from build123d import *

# Parameters (mm, degrees)
SKETCH1_W           = 45.5
SKETCH1_H           = 28.5
BOSS_EXTRUDE1_DEPTH = 14
SKETCH2_R           = 8
CUT_EXTRUDE1_DEPTH  = 30
SKETCH3_R           = 11.1
CUT_EXTRUDE2_DEPTH  = 26
SKETCH4_W           = 9.997259543
SKETCH4_H           = 22.5
CUT_EXTRUDE3_DEPTH  = 56.484231994


with BuildPart() as part:
    # Sketch1 → Boss-Extrude1 (new body)
    with BuildSketch(Plane.XY):
        with Locations((22.75, 14.25)):
            Rectangle(SKETCH1_W, SKETCH1_H)
    extrude(amount=BOSS_EXTRUDE1_DEPTH)

    # Sketch2 → Cut-Extrude1 (cut)
    with BuildSketch(Plane(origin=(0, 28.5, 0), x_dir=(1, 0, 0), z_dir=(0, 1, 0))):
        with Locations((22.75, 0)):
            Circle(SKETCH2_R)
    extrude(amount=-CUT_EXTRUDE1_DEPTH, mode=Mode.SUBTRACT)

    # Sketch3 → Cut-Extrude2 (cut)
    with BuildSketch(Plane.XZ):
        with Locations((22.75, 0)):
            Circle(SKETCH3_R)
    extrude(amount=-CUT_EXTRUDE2_DEPTH, mode=Mode.SUBTRACT)

    # Sketch4 → Cut-Extrude3 (cut, through all)
    with BuildSketch(Plane(origin=(45.5, 0, 0), x_dir=(0, 0, -1), z_dir=(1, 0, 0))):
        with Locations((-4.998629772, 14.75)):
            Rectangle(SKETCH4_W, SKETCH4_H)
    extrude(amount=-CUT_EXTRUDE3_DEPTH, mode=Mode.SUBTRACT)


solid = part.part
The listing builds one solid part. Answer for the finished solid, in the listing's coordinates (mm). A direction names the side the tool comes from. Give positions to 0.01 mm unless a question says otherwise; leave off trailing zeros. Loops run counter-clockwise (first coordinate to the right, second up) from the corner with the lowest first, then second, coordinate; pieces in that order, holes last. Notation, with made-up numbers: M 33,25 L 79,25 A15 ccw 79,50 Z; hole C 0.5,25 d3. An arc over 180 degrees is marked long. Answer as CSV lines item,"result".
Item 1: The part is cut by section B-B (x = 8). Give the vertices of the cut face in (y, z), and give its area (3 significant figures).
Values follow:
outline,"M 0,0 L 3.5,0 L 3.5,10 L 26,10 L 26,0 L 28.5,0 L 28.5,14 L 0,14 Z"
area,"174 mm^2"
Item 2: Which of the six approach directions +Z, -Z, +X, -X, +Y, -Y give full straight-line access (tool end or side, diameter ignored) to faces 1 (the flat face through (39, 3.5, 5)), 2 (the flat face through (0, 14, 12))?
Values follow:
face 1,"-Z, +X, -X"
face 2,"+Z, -Z, -X, +Y, -Y"
Item 3: Straight lines are drawn through the part: line 1 along Y through (x, z) = (7.5, 6.75); line 2 along X through (y, z) = (3.25, 9.25); line 3 along Z through (x, y) = (37, 16). For each, find the intervals that lie inside material, in ascending order. Write a range as [from, to].
Values follow:
line 1,"y = [0, 3.5], [26, 28.5]"
line 2,"x = [0, 16.61], [28.89, 45.5]"
line 3,"z = [10, 14]"
Item 4: The part is cut by section C-C (y = 16). Give the vertices of the cut face in (x, z), and give its area (3 significant figures).
Values follow:
outline,"M 0,10 L 17.93,10 A11.1 cw 27.57,10 L 45.5,10 L 45.5,14 L 0,14 Z"
area,"175 mm^2"
Item 5: The part is cut by section A-A (z = 4.5). Give the vertices of the cut face in (x, y).
Values follow:
outline,"M 0,0 L 12.6,0 L 12.6,3.5 L 0,3.5 Z; M 0,26 L 16.14,26 L 16.14,28.5 L 0,28.5 Z; M 29.36,26 L 45.5,26 L 45.5,28.5 L 29.36,28.5 Z; M 32.9,0 L 45.5,0 L 45.5,3.5 L 32.9,3.5 Z"
Item 6: The part is cut by section D-D (z = 2.25). Give the vertices of the cut face in (x, y), and give its area (3 significant figures).
Values follow:
outline,"M 0,0 L 11.88,0 L 11.88,3.5 L 0,3.5 Z; M 0,26 L 15.07,26 L 15.07,28.5 L 0,28.5 Z; M 30.43,26 L 45.5,26 L 45.5,28.5 L 30.43,28.5 Z; M 33.62,0 L 45.5,0 L 45.5,3.5 L 33.62,3.5 Z"
area,"159 mm^2"
Item 7: Given pin 1 Ø3.5 at (x, z) = (20.5, 7) entering from -Y; pin 2 Ø9 at (x, y) = (35.5, 17) entering from -Z, each flat-ended and moving along its own axis, determine where each tip first touches the part or whether it passes through.
Values follow:
pin 1,"stops at y = 26"
pin 2,"stops at z = 10"
Item 8: The mould has two halves that part along X. Classify faces 3 (the flat face through (22.4, 28.5, 8.5)), 4 (the cylindrical face through (22.994, 9.929, 11.097)), 5 (the cylindrical face through (22.6, 27.3, 8)), 6 (the flat face through (45.5, 14, 12)): released by +X, released by -X, zero draft, split by the parting line, or undercut.
Values follow:
face 3,"zero draft"
face 4,"undercut"
face 5,"undercut"
face 6,"released by +X"
